```python
from build123d import *

# Parameters (mm, degrees)
F0_R     = 3.175
F1_DEPTH = 12.7
F2_DEPTH = 6.35
F3_R     = 0.79375


with BuildPart() as f1:
    # F0 (on Top) → F1 (new body)
    with BuildSketch(Plane.XY):
        Polygon((9.525, -5.499261314), (9.525, 5.499261314), (0, 10.9985226281), (-9.525, 5.499261314), (-9.525, -5.499261314), (0, -10.9985226281), align=None)
        Circle(F0_R, mode=Mode.SUBTRACT)
        Circle(F0_R)
    extrude(amount=F1_DEPTH)

    # F0 (on Top) → F2 (cut)
    with BuildSketch(Plane.XY):
        Circle(F0_R)
    extrude(amount=F2_DEPTH, mode=Mode.SUBTRACT)

    # F3
    f3_edges = [f1.edges().sort_by_distance(p)[0] for p in [
        (0, 10.998523, 6.35),
        (-9.525, 5.499261, 6.35),
        (-4.7625, 8.248892, 0),
        (-4.7625, 8.248892, 12.7),
        (-9.525, -5.499261, 6.35),
        (-9.525, 0, 0),
        (-9.525, 0, 12.7),
        (0, -10.998523, 6.35),
        (-4.7625, -8.248892, 0),
        (-4.7625, -8.248892, 12.7),
        (9.525, -5.499261, 6.35),
        (4.7625, -8.248892, 0),
        (4.7625, -8.248892, 12.7),
        (9.525, 0, 12.7),
        (4.7625, 8.248892, 12.7),
        (9.525, 5.499261, 6.35),
        (9.525, 0, 0),
        (4.7625, 8.248892, 0),
        (3.175, 0, 3.175),
        (-3.175, 0, 0),
        (-3.175, 0, 6.35),
    ]]
    fillet(f3_edges, radius=F3_R)


solid = f1.part
```
For this review, take the finished solid that the model builds, in its own axes (mm). Round coordinates to 2 decimals unless told otherwise and drop trailing zeros. Loops run counter-clockwise (first coordinate to the right, second up) from the corner with the lowest first, then second, coordinate; pieces in that order, holes last.
(1) Wall thickness on line 1 along Y through (x, z) = (0, 2.95) (3 decimals); line 2 along X through (y, z) = (-1, 5.75) (3 decimals); line 3 along Y through (x, z) = (-1.5, 4.5): over which ranges is each line inside the solid? List them lowest first.
Returned:
line 1: y = -10.876 to -3.175, 3.175 to 10.876
line 2: x = -9.525 to -2.988, 2.988 to 9.525
line 3: y = -10.13 to -2.8, 2.8 to 10.13
(2) We need section C-C (z = 11). Give the boundary of the cut face in (x, y) (1 decimal).
Returned:
outline: (-9.5, -5) arc R0.8 ccw to (-9.1, -5.7) - (-0.4, -10.8) arc R0.8 ccw to (0.4, -10.8) - (9.1, -5.7) arc R0.8 ccw to (9.5, -5) - (9.5, 5) arc R0.8 ccw to (9.1, 5.7) - (0.4, 10.8) arc R0.8 ccw to (-0.4, 10.8) - (-9.1, 5.7) arc R0.8 ccw to (-9.5, 5) - close
(3) Clearance check with flat-ended pins moving along their axes: P1, Ø4, axis at x = -4, z = 7, coming from the +Y side; P2, Ø1.5, axis at x = -5.5, y = 8, coming from the +Z side; P3, Ø1.5, axis at x = -3, z = 4.5, coming from the -Y side. State where each tip first meets the part, or that it passes through.
Returned:
P1: stops at y = 9.84
P2: stops at z = 12.68
P3: stops at y = -9.7
(4) Mouldability with a two-part tool opening along Y and no side actions: class faces 1 (the cylindrical face through (-0.69, -3.1, 3.14)), 2 (the flat face through (0, 0, 6.35)), 3 (the cylindrical face through (4.59, 8.09, 0.24)), 4 (the flat face through (-0.1, -4.3, 0)) as released by +Y, released by -Y, zero draft, split by the parting line, or undercut.
Returned:
face 1: undercut
face 2: undercut
face 3: released by +Y
face 4: zero draft
